Can you work these out from the model? Positions are in its coordinate system, mm. Face numbers are marked on the shaded views. A direction names the side the tool comes from. Give positions to 0.01 mm unless a question says otherwise; leave off trailing zeros. Write each loop counter-clockwise with the first axis right and the second up, starting at its lowest first coordinate (ties: lowest second). Pieces come first, ordered by that corner, then holes. Notation, with made-up numbers: (66.5, 28.25) -> (105.5, 28.25) arc R24 ccw to (105.5, 48.25) -> close; hole circle Ø8 at (56.5, -18). An arc over 180 degrees is marked (long way). Answer as CSV lines item,"result". Start each with the question number.
1. I'm going to push flat-ended pins straight in: P1, Ø2, axis at x = 5.5, z = 2, coming from the +Y side; P2, Ø3, axis at x = 12, y = 1, coming from the +Z side; P3, Ø3, axis at y = 4, z = -2, coming from the -X side. Where does each tip first touch, or does it pass through?
2. I need wall thicknesses on line 1 (Z direction, x = 14.25, y = 0); line 2 (X direction, y = -0.75, z = -2); line 3 (X direction, y = -1.25, z = 4.5). Which ranges of each line are inside material? Lowest first, please. Write a range as [from, to].
3. If we section it at A-A on x = 14.5: Write out the boundary of the cut face in (y, z), plus the area to 3 significant figures.
4. On a 3-axis mill with a long thin cutter (end or side, diameter ignored), from which of +Z, -Z, +X, -X, +Y, -Y can I reach the whole of each face in a straight line? I mean the marked faces 1 and 2. Say none if no direction works.
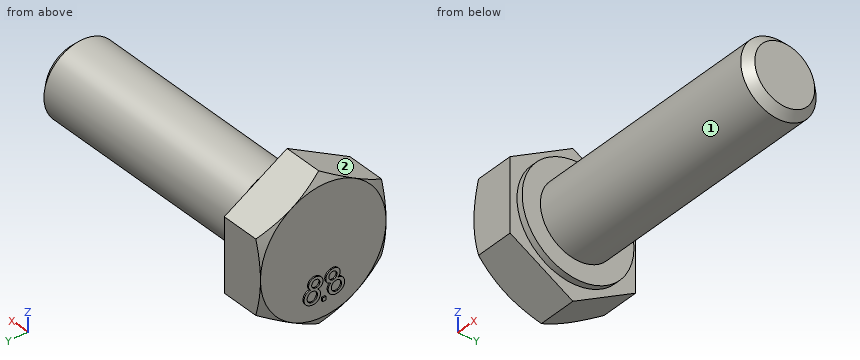
Autodesk Inventor part; units mm, degrees
ref_plane "YZ Plane" through (0, 0, 0) normal (1, 0, 0) x (0, 1, 0)
ref_plane "XZ Plane" through (0, 0, 0) normal (0, 1, 0) x (-1, 0, 0)
ref_plane "XY Plane" through (0, 0, 0) normal (0, 0, 1) x (1, 0, 0)
sketch "Sketch1" plane through (0, 0, 0) normal (0, 0, 1) x (1, 0, 0)
  line L0 (-8.8, 0) -> (24.8, 0)
  line L1 (20, 0) -> (20, 2.385)
  line L2 (20, 2.385) -> (19.385, 3)
  line L3 (19.385, 3) -> (0, 3)
  line L4 (0, 3) -> (0, 4.45)
  line L5 (0, 4.45) -> (-0.5, 4.45)
  line L6 (-0.5, 4.45) -> (-0.5, 5)
  line L7 (-0.5, 5) -> (-4, 5)
  line L8 (-4, 5) -> (-4, 0)
  point P0 (0, 0)
  dimension "d0" = 6
  dimension "d1" = 20
  dimension "d2" = 10
  dimension "d3" = 8.9
  dimension "d4" = 4
  dimension "d5" = 45
  dimension "d6" = 4.77
  dimension "d7" = 0.5
revolve "Revolution1" add sketch "Sketch1" angle 360 about axis through (-10, 0, 0) along (1, 0, 0)
sketch "Sketch2" plane through (-4, 0, 0) normal (-1, 0, 0) x (0, 0, 1)
  circle A0 centre (0, 0) radius 5
  line L0 (2.8868, 5) -> (5.7735, 0)
  line L1 (5.7735, 0) -> (2.8868, -5)
  line L2 (2.8868, -5) -> (-2.8868, -5)
  line L3 (-2.8868, -5) -> (-5.7735, 0)
  line L4 (-5.7735, 0) -> (-2.8868, 5)
  line L5 (-2.8868, 5) -> (2.8868, 5)
  point P0 (0, 5)
extrude "Extrusion1" add sketch "Sketch2" against normal up to surface (3.5 mm away)
sketch "Sketch3" plane through (0, 0, 0) normal (0, 0, 1) x (1, 0, 0)
  line L0 (-4, 5.55) -> (-0.5, 5.55)
  line L1 (-0.5, 5.55) -> (-0.5, 6.66)
  line L2 (-0.5, 6.66) -> (-4, 6.66)
  line L3 (-4, 6.66) -> (-4, 5.55)
  line L4 (-4.8, 0) -> (0.8, 0)
  line L5 (-4, 5) -> (-3.0416, 6.66)
  line L6 (-4, 5.55) -> (-4, 5)
  point P0 (0, 0)
  point P1 (-0.5, 5)
  dimension "d11" = 11.1
  dimension "d12" = 1.11
  dimension "d13" = 30
revolve "Revolution2" cut sketch "Sketch3" angle 360 about axis through (-10, 0, 0) along (1, 0, 0) contours L3 L2 L5 L0 | L0 L5 L6
thread "Thread1"
sketch "Sketch4" plane through (-4, 0, 0) normal (-1, 0, 0) x (0, 0, 1)
  circle A0 centre (0, 0) radius 3.75 construction
  spline S0 degree 2 poles (-2.4547, -1.0741) (-2.3544, -1.2038) (-2.112, -1.282) (-1.9755, -1.2387) knots 0 0 0 1 2 2 2
  spline S1 degree 2 poles (-1.9755, -1.2387) (-1.7677, -1.1728) (-1.5794, -0.7835) (-1.6577, -0.5365) knots 0 0 0 1 2 2 2
  spline S2 degree 2 poles (-1.6577, -0.5365) (-1.7371, -0.2866) (-2.1226, -0.0747) (-2.3304, -0.1406) knots 0 0 0 1 2 2 2
  spline S3 degree 2 poles (-2.3304, -0.1406) (-2.4626, -0.1826) (-2.6145, -0.3843) (-2.623, -0.5438) knots 0 0 0 1 2 2 2
  spline S4 degree 2 poles (-2.623, -0.5438) (-2.736, -0.3845) (-3.0498, -0.2826) (-3.227, -0.3389) knots 0 0 0 1 2 2 2
  spline S5 degree 2 poles (-3.227, -0.3389) (-3.4711, -0.4163) (-3.6941, -0.8677) (-3.6047, -1.1496) knots 0 0 0 1 2 2 2
  spline S6 degree 2 poles (-3.6047, -1.1496) (-3.5152, -1.4315) (-3.0713, -1.6712) (-2.8214, -1.5919) knots 0 0 0 1 2 2 2
  spline S7 degree 2 poles (-2.8214, -1.5919) (-2.6354, -1.5329) (-2.444, -1.2642) (-2.4547, -1.0741) knots 0 0 0 1 2 2 2
  spline S8 degree 2 poles (-2.8994, -1.3512) (-2.9996, -1.383) (-3.217, -1.348) (-3.3792, -1.1948) (-3.4133, -1.0873) knots 0 0 0 1 2 3 3 3
  spline S9 degree 2 poles (-3.4133, -1.0873) (-3.4668, -0.9187) (-3.319, -0.6335) (-3.1534, -0.581) knots 0 0 0 1 2 2 2
  spline S10 degree 2 poles (-3.1534, -0.581) (-2.9834, -0.527) (-2.6915, -0.6807) (-2.638, -0.8492) knots 0 0 0 1 2 2 2
  spline S11 degree 2 poles (-2.638, -0.8492) (-2.5855, -1.0149) (-2.7352, -1.2991) (-2.8994, -1.3512) knots 0 0 0 1 2 2 2
  spline S12 degree 2 poles (-2.0433, -0.9947) (-2.1784, -1.0376) (-2.4047, -0.9191) (-2.4486, -0.7811) knots 0 0 0 1 2 2 2
  spline S13 degree 2 poles (-2.4486, -0.7811) (-2.4914, -0.646) (-2.3759, -0.4206) (-2.2524, -0.3814) knots 0 0 0 1 2 2 2
  spline S14 degree 2 poles (-2.2524, -0.3814) (-2.1245, -0.3408) (-1.8929, -0.4608) (-1.8509, -0.593) knots 0 0 0 1 2 2 2
  spline S15 degree 2 poles (-1.8509, -0.593) (-1.808, -0.7282) (-1.9242, -0.9569) (-2.0433, -0.9947) knots 0 0 0 1 2 2 2
  line L0 (-3.75, -0.1349) -> (-3.471, -0.1349)
  line L1 (-3.471, -0.1349) -> (-3.471, 0.1441)
  line L2 (-3.471, 0.1441) -> (-3.75, 0.1441)
  line L3 (-3.75, 0.1441) -> (-3.75, -0.1349)
  spline S16 degree 2 poles (-2.6249, 0.538) (-2.6177, 0.3742) (-2.4648, 0.1705) (-2.3282, 0.1272) knots 0 0 0 1 2 2 2
  spline S17 degree 2 poles (-2.3282, 0.1272) (-2.1205, 0.0612) (-1.7421, 0.2706) (-1.6637, 0.5176) knots 0 0 0 1 2 2 2
  spline S18 degree 2 poles (-1.6637, 0.5176) (-1.5844, 0.7675) (-1.7772, 1.163) (-1.985, 1.2289) knots 0 0 0 1 2 2 2
  spline S19 degree 2 poles (-1.985, 1.2289) (-2.1172, 1.2709) (-2.3576, 1.1936) (-2.4566, 1.0683) knots 0 0 0 1 2 2 2
  spline S20 degree 2 poles (-2.4566, 1.0683) (-2.457, 1.2636) (-2.6546, 1.5278) (-2.8319, 1.5841) knots 0 0 0 1 2 2 2
  spline S21 degree 2 poles (-2.8319, 1.5841) (-3.076, 1.6615) (-3.5184, 1.4213) (-3.6079, 1.1394) knots 0 0 0 1 2 2 2
  spline S22 degree 2 poles (-3.6079, 1.1394) (-3.6973, 0.8576) (-3.4729, 0.4057) (-3.223, 0.3264) knots 0 0 0 1 2 2 2
  spline S23 degree 2 poles (-3.223, 0.3264) (-3.037, 0.2674) (-2.7257, 0.3765) (-2.6249, 0.538) knots 0 0 0 1 2 2 2
  spline S24 degree 2 poles (-3.1479, 0.568) (-3.2482, 0.5999) (-3.4056, 0.7538) (-3.4498, 0.9725) (-3.4156, 1.08) knots 0 0 0 1 2 3 3 3
  spline S25 degree 2 poles (-3.4156, 1.08) (-3.3621, 1.2486) (-3.0769, 1.3963) (-2.9113, 1.3438) knots 0 0 0 1 2 2 2
  spline S26 degree 2 poles (-2.9113, 1.3438) (-2.7413, 1.2898) (-2.5915, 0.996) (-2.645, 0.8274) knots 0 0 0 1 2 2 2
  spline S27 degree 2 poles (-2.645, 0.8274) (-2.6975, 0.6618) (-2.9837, 0.5159) (-3.1479, 0.568) knots 0 0 0 1 2 2 2
  spline S28 degree 2 poles (-2.243, 0.3656) (-2.3781, 0.4085) (-2.4947, 0.6358) (-2.4509, 0.7738) knots 0 0 0 1 2 2 2
  spline S29 degree 2 poles (-2.4509, 0.7738) (-2.408, 0.909) (-2.1836, 1.0265) (-2.0601, 0.9873) knots 0 0 0 1 2 2 2
  spline S30 degree 2 poles (-2.0601, 0.9873) (-1.9322, 0.9467) (-1.8122, 0.7151) (-1.8542, 0.5829) knots 0 0 0 1 2 2 2
  spline S31 degree 2 poles (-1.8542, 0.5829) (-1.897, 0.4477) (-2.1238, 0.3278) (-2.243, 0.3656) knots 0 0 0 1 2 2 2
  dimension "d17" = 7.5
extrude "Extrusion2" add sketch "Sketch4" along normal blind 0.1
equation "\"d7\" = 0.125 * d4"
equation "\"d12\" = 0.1 * d11"
properties part number "Sechskantschraube ISO 4017-M6x20-8.8" material "Steel"
Computed values:
1,P1,"stops at y = 2.83"
1,P2,"stops at z = 3"
1,P3,"stops at x = -4"
2,line 1,"z = [-3, 3]"
2,line 2,"x = [-4, 20]"
2,line 3,"x = [-4, -0.5]"
3,outline,"circle Ø6 at (0, 0)"
3,area,"28.3 mm2"
4,face 1,"+X"
4,face 2,"+Z, +X, -X, -Y"
